Work out the finished part from the listing and answer in its coordinate system (mm). A direction names the side the tool comes from. Round coordinates to 2 decimals unless told otherwise and drop trailing zeros. Write each loop counter-clockwise with the first axis right and the second up, starting at its lowest first coordinate (ties: lowest second). Pieces come first, ordered by that corner, then holes. Notation, with made-up numbers: M -6,59.25 L 6,59.25 A19 cw 6,78.25 Z; hole C -12.75,-36.75 d10. An arc over 180 degrees is marked long. Answer in a Markdown table with one row per item.
```python
from build123d import *

# Parameters (mm, degrees)
F2_DEPTH = 25


with BuildPart() as f2:
    # F1 (on face) → F2 (new body)
    with BuildSketch(Plane.YZ):
        Polygon((-55.588484, -44.88135), (55.588484, -44.88135), (0, 51.400729), align=None)
        Polygon((51.258357, -42.38135), (-51.258357, -42.38135), (0, 46.400729), align=None, mode=Mode.SUBTRACT)
    extrude(amount=F2_DEPTH)


solid = f2.part
```
1. Determine the mould class of faces 1 (the flat face through (12.32, 25.27, 2.63)), 2 (the flat face through (12.325, -25.988, 1.388)), 3 (the flat face through (12, -1, -44.881)), 4 (the flat face through (12.32, 28.18, 2.59)) for opening direction Z: released by +Z, released by -Z, zero draft, split by the parting line, or undercut.
Calculated:
| item | result |
|---|---|
| face 1 | undercut |
| face 2 | undercut |
| face 3 | released by -Z |
| face 4 | released by +Z |
2. The part is cut by section B-B (y = -16). Determine the outline of the cut face in (x, z).
Calculated:
| item | result |
|---|---|
| outline | M 0,-44.88 L 25,-44.88 L 25,-42.38 L 0,-42.38 Z; M 0,18.69 L 25,18.69 L 25,23.69 L 0,23.69 Z |
3. Given pin 1 (12.5 mm diameter, centred on x = 18.5, y = -22, fed in from +Z); pin 2 (1.5 mm diameter, centred on x = 15, y = -41, fed in from +Z); pin 3 (8 mm diameter, centred on x = 6, z = 29, fed in from +Y); pin 4 (8 mm diameter, centred on y = 22, z = -4.5, fed in from +X), each flat-ended and moving along its own axis, determine where each tip first touches the part or whether it passes through.
Calculated:
| item | result |
|---|---|
| pin 1 | stops at z = 24.12 |
| pin 2 | stops at z = -18.31 |
| pin 3 | stops at y = 15.24 |
| pin 4 | passes through |
4. Consider line 1 along Y through (x, z) = (12.5, -31); line 2 along Z through (x, y) = (1.75, 14.5); line 3 along Y through (x, z) = (13, 31.5). Determine where each line is inside the solid, lowest interval first. Write a range as from..to.
Calculated:
| item | result |
|---|---|
| line 1 | y = -47.57..-44.69, 44.69..47.57 |
| line 2 | z = -44.88..-42.38, 21.29..26.29 |
| line 3 | y = -11.49..-8.6, 8.6..11.49 |
5. A tool of negligible diameter and unlimited length cuts with its end or side. For faces 5 (the flat face through (12, 1, -42.381)), 6 (the flat face through (12.325, -27.405, 3.934)), from which of +Z, -Z, +X, -X, +Y, -Y can it reach the whole face along a straight path? Write none if from no direction.
Calculated:
| item | result |
|---|---|
| face 5 | +X, -X |
| face 6 | +Z, +X, -X, -Y |
6. The part is cut by section A-A (x = 18). Determine the outline of the cut face in (y, z), plus the area to 3 significant figures.
Calculated:
| item | result |
|---|---|
| outline | M -55.59,-44.88 L 55.59,-44.88 L 0,51.4 Z; hole M -51.26,-42.38 L 51.26,-42.38 L 0,46.4 Z |
| area | 801 mm² |
7. The part is cut by section C-C (z = 16). Determine the outline of the cut face in (x, y), plus the area to 3 significant figures.
Calculated:
| item | result |
|---|---|
| outline | M 0,-20.44 L 25,-20.44 L 25,-17.55 L 0,-17.55 Z; M 0,17.55 L 25,17.55 L 25,20.44 L 0,20.44 Z |
| area | 144 mm² |
